Geometry: final body of the model. Coordinates: model frame, mm. Face numbers are marked on the shaded views. A direction names the side the tool comes from. Coordinates: 2 decimals unless noted, no trailing zeros. Loops run counter-clockwise (first coordinate to the right, second up) from the corner with the lowest first, then second, coordinate; pieces in that order, holes last. Notation, with made-up numbers: (46, -20) - (65, -20) arc R16 ccw to (65, -3) - close; hole circle Ø4 at (75, -31.75). An arc over 180 degrees is marked (long way). Return JSON: item names as keys, results as strings.
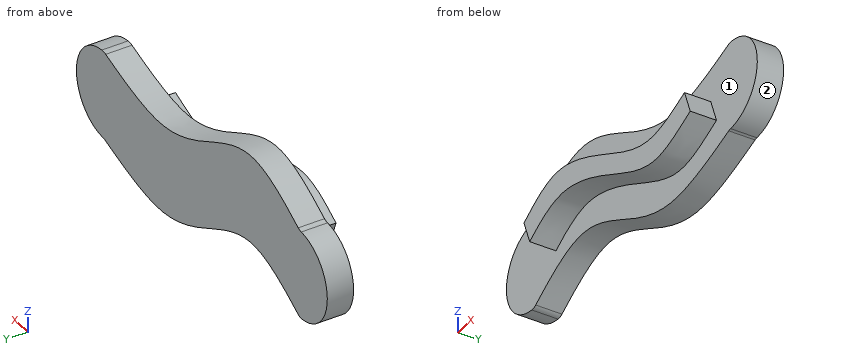
from build123d import *

# Parameters (mm, degrees)
F1_DEPTH = 12.7
F2_DEPTH = 25.4
F3_R     = 7.62
F4_R     = 5.08
F5_R     = 5.08
F6_R     = 5.08


# Not quite as in the source:
# - the program builds the solid bodies; features that only make, move or delete a surface that nothing else refers to are left out


with BuildPart() as f1:
    # F0 (on Front) → F1 (new body)
    with BuildSketch(Plane.XZ):
        with BuildLine():
            add(Edge.make_bspline(
                [(-76.5334740281, 20.7332828829), (-63.8515293548, 28.3869740492), (-38.487641079, 43.6943557355), (-0.1074870643, 19.2987869132), (33.6920782855, 6.372177087), (61.7287419774, 15.7705051868), (76.5334740281, 20.7332828829)],
                knots=[0, 0, 0, 0, 0.252598913, 0.5051978047, 0.7387201987, 1, 1, 1, 1], degree=3))
            Line((-76.5334740281, 20.7332828829), (-76.5334740281, -22.4467171171))
            add(Edge.make_bspline(
                [(-76.5334740281, -22.4467171171), (-63.8515293548, -14.7930259508), (-38.487641079, 0.5143557355), (-0.1074870643, -23.8812130868), (33.6920782855, -36.807822913), (61.7287419774, -27.4094948132), (76.5334740281, -22.4467171171)],
                knots=[0, 0, 0, 0, 0.252598913, 0.5051978047, 0.7387201987, 1, 1, 1, 1], degree=3))
            Line((76.5334740281, -22.4467171171), (76.5334740281, 20.7332828829))
        make_face()
        with BuildLine():
            Line((-59.3705394858, -3.9110629208), (-63.8515293548, 7.9721491784))
            add(Edge.make_bspline(
                [(-63.8515293548, 7.9721491784), (-55.8466582979, 13.0095149676), (-38.1452218943, 24.1488087208), (0.3419863459, 5.213337181), (32.9615149645, -12.272359942), (52.4893434663, -3.9416111996), (61.7287419774, 0)],
                knots=[0, 0, 0, 0, 0.228361581, 0.5049835251, 0.7657878611, 1, 1, 1, 1], degree=3))
            Line((61.7287419774, 0), (66.2097318464, -11.8832120992))
            add(Edge.make_bspline(
                [(-59.3705394858, -3.9110629208), (-51.3634228426, 1.1277159879), (-33.1115500983, 10.7952182475), (5.0660805533, -7.2965458084), (37.9471343056, -25.5812525078), (56.9802173789, -15.8206066761), (66.2097318464, -11.8832120992)],
                knots=[0, 0, 0, 0, 0.2284256427, 0.505143577, 0.7660384145, 1, 1, 1, 1], degree=3))
        make_face(mode=Mode.SUBTRACT)
        with BuildLine():
            Line((-76.5334740281, -22.4467171171), (-76.5334740281, 20.7332828829))
            ThreePointArc((-76.5334740281, 20.7332828829), (-98.1234740281, -0.8567171171), (-76.5334740281, -22.4467171171))
        make_face()
        with BuildLine():
            ThreePointArc((76.5334740281, -22.4467171171), (98.1234740281, -0.8567171171), (76.5334740281, 20.7332828829))
            Line((76.5334740281, 20.7332828829), (76.5334740281, -22.4467171171))
        make_face()
    extrude(amount=F1_DEPTH)

    # F0 (on Front) → F2 (join)
    with BuildSketch(Plane.XZ):
        with BuildLine():
            add(Edge.make_bspline(
                [(-63.8515293548, 7.9721491784), (-55.8466582979, 13.0095149676), (-38.1452218943, 24.1488087208), (0.3419863459, 5.213337181), (32.9615149645, -12.272359942), (52.4893434663, -3.9416111996), (61.7287419774, 0)],
                knots=[0, 0, 0, 0, 0.228361581, 0.5049835251, 0.7657878611, 1, 1, 1, 1], degree=3))
            Line((-63.8515293548, 7.9721491784), (-59.3705394858, -3.9110629208))
            add(Edge.make_bspline(
                [(-59.3705394858, -3.9110629208), (-51.3634228426, 1.1277159879), (-33.1115500983, 10.7952182475), (5.0660805533, -7.2965458084), (37.9471343056, -25.5812525078), (56.9802173789, -15.8206066761), (66.2097318464, -11.8832120992)],
                knots=[0, 0, 0, 0, 0.2284256427, 0.505143577, 0.7660384145, 1, 1, 1, 1], degree=3))
            Line((66.2097318464, -11.8832120992), (61.7287419774, 0))
        make_face()
    extrude(amount=F2_DEPTH)

    # F3
    f3_edges = [f1.edges().sort_by_distance(p)[0] for p in [
        (76.533474, -6.35, 20.733283),
    ]]
    fillet(f3_edges, radius=F3_R)

    # F4
    f4_edges = [f1.edges().sort_by_distance(p)[0] for p in [
        (-76.533474, -6.35, -22.446717),
    ]]
    fillet(f4_edges, radius=F4_R)

    # F5
    f5_edges = [f1.edges().sort_by_distance(p)[0] for p in [
        (-76.533474, -6.35, 20.733283),
    ]]
    fillet(f5_edges, radius=F5_R)

    # F6
    f6_edges = [f1.edges().sort_by_distance(p)[0] for p in [
        (76.533474, -6.35, -22.446717),
    ]]
    fillet(f6_edges, radius=F6_R)


solid = f1.part
Item 1: Section query A-A, the plane x = -81. Return loops of the section in (y, z).
Worked out:
{"outline": "(-12.7, -21.98) - (0, -21.98) - (0, 20.27) - (-12.7, 20.27) - close"}
Item 2: Ray query, probe 1 along Y at (x, z) = (32.5, -24.5); probe 2 along X at (y, z) = (-18, 1); probe 3 along Z at (x, y) = (72.5, -7.25). Return the intervals inside material, ascending. Write a range as from..to.
Worked out:
{"probe 1": "-12.7..0", "probe 2": "-61.22..-50.77, -13.86..8.08", "probe 3": "-23.8..19.38"}
Item 3: First-contact query: pin 1 Ø4 at (x, z) = (49.5, 6.5) entering from -Y; pin 2 Ø10 at (x, y) = (-0.5, -4.5) entering from -Z; pin 3 Ø5 at (y, z) = (-6.5, -18.5) entering from +X. Flat tips, straight axial feed; report the tip coordinate or a pass-through.
Worked out:
{"pin 1": "y = -12.7", "pin 2": "z = -24.67", "pin 3": "x = 91.92"}
Item 4: Reachability of the marked faces 1 and 2 from +Z, -Z, +X, -X, +Y, -Y: full face, straight path, thin tool, end or side. Return the list, or none.
Worked out:
{"face 1": "-Y", "face 2": "+X, +Y, -Y"}
